```python
from build123d import *

# Parameters (mm, degrees)
BOSS_EXTRUDE1_DEPTH = 10
CUT_EXTRUDE1_DEPTH  = 6


with BuildPart() as part:
    # Sketch1 → Boss-Extrude1 (new body)
    with BuildSketch(Plane(origin=(0, 0, 0), x_dir=(1, 0, 0), z_dir=(0, 1, 0))):
        with BuildLine():
            Line((0.309633028, -3.737195123), (16.548165138, -2.391804879))
            ThreePointArc((16.548165138, -2.391804879), (18.75, 0), (16.548165138, 2.391804879))
            Line((16.548165138, 2.391804879), (0.309633028, 3.737195123))
            ThreePointArc((0.309633028, 3.737195123), (-3.75, 0), (0.309633028, -3.737195123))
        make_face()
    extrude(amount=BOSS_EXTRUDE1_DEPTH)

    # Sketch2 → Cut-Extrude1 (cut)
    with BuildSketch(Plane(origin=(0, 10, 0), x_dir=(1, 0, 0), z_dir=(0, 1, 0))):
        with BuildLine():
            Line((-1.67, -1.887193684), (-1.67, -5.52))
            Line((-1.67, -5.52), (1.67, -5.52))
            Line((1.67, -5.52), (1.67, -1.887193684))
            ThreePointArc((1.67, -1.887193684), (2.52, 0), (1.67, 1.887193684))
            Line((1.67, 1.887193684), (1.67, 5.52))
            Line((1.67, 5.52), (-1.67, 5.52))
            Line((-1.67, 5.52), (-1.67, 1.887193684))
            ThreePointArc((-1.67, 1.887193684), (-2.52, 0), (-1.67, -1.887193684))
        make_face()
    extrude(amount=-CUT_EXTRUDE1_DEPTH, mode=Mode.SUBTRACT)


solid = part.part
```
The listing builds one solid part. Answer for the finished solid, in the listing's coordinates (mm). A direction names the side the tool comes from. Round coordinates to 2 decimals unless told otherwise and drop trailing zeros. Order: outer loops, then holes, each group sorted by start corner. A loop starts at its lowest first (then second) coordinate and runs counter-clockwise, first axis right, second up. Notation, with made-up numbers: (-22.5, 42.5) - (-1.5, 42.5) arc R4 ccw to (-1.5, 47.5) - close; hole circle Ø5 at (49, 10.25). An arc over 180 degrees is marked (long way). Put each result on its own line as item: value. Start each with the question number.
(1) Find section C-C (y = 3.5). Give the vertices of the cut face in (x, z).
(2) For faces 4 (the flat face through (7, 0, 0)), 5 (the cylindrical face through (-2.52, 7.04, -0.03)), 6 (the flat face through (-1.67, 7, -3)), determine the directions among +Z, -Z, +X, -X, +Y, -Y from which every point of the face is accessible in a straight line to the end or side of a thin tool.
(3) Determine the mould class of faces 1 (the flat face through (1.67, 7, -3)), 2 (the cylindrical face through (18.75, 4.93, 0.05)), 3 (the flat face through (10, 10, 0)) for opening direction X: released by +X, released by -X, zero draft, split by the parting line, or undercut.
(4) Find section D-D (z = 1). Give the vertices of the cut face in (x, y).
(5) Find section B-B (x = 0). Give the vertices of the cut face in (y, z), plus the area to 3 significant figures.
(6) Given P1, Ø2.5, axis at x = 0, z = -1, coming from the +Y side; P2, Ø1, axis at x = 15.5, y = 6, coming from the -Z side; P3, Ø1.4, axis at y = 8, z = 3, coming from the -X side, each flat-ended and moving along its own axis, determine where each tip first touches the part or whether it passes through.
(7) Straight lines are drawn through the part: probe 1 along X at (y, z) = (7, 1); probe 2 along X at (y, z) = (5, 1.25); probe 3 along Z at (x, y) = (5.5, 2.25). For each, find the intervals that lie inside material, in ascending order. Write a range as from..to.
(8) Find section A-A (z = 0). Give the vertices of the cut face in (x, y).
Reply:
1. outline: (0.31, -3.74) - (16.55, -2.39) arc R2.4 ccw to (16.55, 2.39) - (0.31, 3.74) arc R3.75 ccw (long way) to start
2. face 4: +Z, -Z, +X, -X, -Y
2. face 5: +Y
2. face 6: +Z, -Z, +Y
3. face 1: undercut
3. face 2: released by +X
3. face 3: zero draft
4. outline: (-3.61, 0) - (18.53, 0) - (18.53, 10) - (2.31, 10) - (2.31, 4) - (-2.31, 4) - (-2.31, 10) - (-3.61, 10) - close
5. outline: (0, -3.75) - (4, -3.75) - (4, 3.75) - (0, 3.75) - close
5. area: 30.0 mm^2
6. P1: y = 4
6. P2: z = -2.52
6. P3: x = -2.96
7. probe 1: -3.61..-2.31, 2.31..18.53
7. probe 2: -3.54..-2.19, 2.19..18.4
7. probe 3: -3.31..3.31
8. outline: (-3.75, 0) - (18.75, 0) - (18.75, 10) - (2.52, 10) - (2.52, 4) - (-2.52, 4) - (-2.52, 10) - (-3.75, 10) - close
